Here's how the part is built. I have some questions about the finished solid (model axes, mm). A direction names the side the tool comes from. Round coordinates to 2 decimals unless told otherwise and drop trailing zeros. Write each loop counter-clockwise with the first axis right and the second up, starting at its lowest first coordinate (ties: lowest second). Pieces come first, ordered by that corner, then holes. Notation, with made-up numbers: (7.5, 77) -> (45.5, 77) arc R28 cw to (45.5, 104) -> close; hole circle Ø6 at (68, 74.25). An arc over 180 degrees is marked (long way). Put each result on its own line as item: value. Start each with the question number.
1) I want a section at B-B, the plane z = 46.99. List the corners of the cut face in (x, y) for me, then the cut area to 3 significant figures.
2) I want a section at D-D, the plane z = -16.51. Give the number of separate pieces and of enclosed holes in the cut face, then the cut area to 3 significant figures.
3) Will these pins go through, and if not, where does the flat tip stop? P1, Ø12, axis at y = 80.5, z = 34.5, coming from the -X side; P2, Ø0.9, axis at x = 1, z = 32.5, coming from the -Y side; P3, Ø0.8, axis at x = 1, z = 42.5, coming from the -Y side.
4) If I drill on line 1 along Y through (x, z) = (0.9, 46.99); line 2 along Y through (x, z) = (0.5, -18); line 3 along Y through (x, z) = (-3.25, 13.5), over which ranges is the centre line in solid material (lowest first)? Write a range as [from, to].
5) I want a section at C-C, the plane y = 12.7. List the corners of the cut face in (x, z) for me, then the cut area to 3 significant figures.
6) Which directions (+Z, -Z, +X, -X, +Y, -Y) give clear straight access to the entire face, cutting with the end or side of a thin tool? Please do faces 1 (the cylindrical face through (-0.955, 2.493, -4.952)), 2 (the flat face through (0.783, 25.561, -17.647)), 3 (the flat face through (-7, 1, 31.75)), 4 (the cylindrical face through (-11.62, 0.8, -2.73)), 5 (the cylindrical face through (0.2, 1.4, -5)).
7) I want a section at A-A, the plane y = 107.95. List the corners of the cut face in (x, z) for me, then the cut area to 3 significant figures.
8) We'd pull the mould along Z, two halves only. Please class faces 6 (the cylindrical face through (-12.943, 0.805, 17.205)), 7 (the flat face through (0.783, 46.246, 17.647)), 8 (the flat face through (0.3, 59.3, -40.64)), 9 (the cylindrical face through (0.805, 119.926, 30.986)): released by +Z, released by -Z, zero draft, split by the parting line, or undercut.
from build123d import *

# Parameters (mm, degrees)
SKETCH2_R                     = 14.2875
SKETCH2_R_2                   = 2.54
BOSS_EXTRUDE1_DEPTH           = 1.5875
SKETCH7_W                     = 1.5875
SKETCH7_H                     = 27.94
CUT_EXTRUDE1_DEPTH            = 0.00254
EDGE_FLANGE2_STRIP_W          = 12.7
EDGE_FLANGE2_STRIP_H          = 1.5875
EDGE_FLANGE2_STRIP_CUT_DEPTH  = 72.39
EDGE_FLANGE2_RELIEF_W         = 13.49375
EDGE_FLANGE2_RELIEF_H         = 0.79375
EDGE_FLANGE2_RELIEF_CUT_DEPTH = 1.5875
EDGE_FLANGE2_DEPTH            = 72.39
SKETCH14_R                    = 2.54
CUT_EXTRUDE2_DEPTH            = 1.5875
FILLET1_R                     = 2.54


# Sheet-metal steps are written as plain solids
with BuildPart() as part:
    # Sketch2 → Boss-Extrude1 (new body)
    with BuildSketch(Plane(origin=(0, 0, 0), x_dir=(0, 0, -1), z_dir=(1, 0, 0))):
        Polygon((-59.69, 95.25), (-59.69, 0), (40.64, 0), (40.64, 95.25), (40.64, 120.65), (-31.75, 120.65), (-31.75, 95.25), align=None)
        with Locations((0, 80.264)):
            Circle(SKETCH2_R, mode=Mode.SUBTRACT)
        with Locations((-46.99, 80.264)):
            Circle(SKETCH2_R_2, mode=Mode.SUBTRACT)
        with Locations((-46.99, 63.373)):
            Circle(SKETCH2_R_2, mode=Mode.SUBTRACT)
        with Locations((-17.272, 107.95)):
            Circle(SKETCH2_R_2, mode=Mode.SUBTRACT)
        with Locations((-2.794, 107.95)):
            Circle(SKETCH2_R_2, mode=Mode.SUBTRACT)
        with Locations((11.684, 107.95)):
            Circle(SKETCH2_R_2, mode=Mode.SUBTRACT)
        with Locations((26.162, 107.95)):
            Circle(SKETCH2_R_2, mode=Mode.SUBTRACT)
        with Locations((-46.99, 46.482)):
            Circle(SKETCH2_R_2, mode=Mode.SUBTRACT)
        with Locations((-46.99, 29.591)):
            Circle(SKETCH2_R_2, mode=Mode.SUBTRACT)
        with Locations((-46.99, 12.7)):
            Circle(SKETCH2_R_2, mode=Mode.SUBTRACT)
        with BuildLine():
            Line((-27.305, 64.866068321), (-8.255, 53.867545693))
            ThreePointArc((-8.255, 53.867545693), (-7.62, 52.76769343), (-8.255, 51.667841167))
            Line((-8.255, 51.667841167), (-27.305, 40.669318539))
            ThreePointArc((-27.305, 40.669318539), (-28.575, 40.669318539), (-29.21, 41.769170802))
            Line((-29.21, 41.769170802), (-29.21, 63.766216058))
            ThreePointArc((-29.21, 63.766216058), (-28.575, 64.866068321), (-27.305, 64.866068321))
        make_face(mode=Mode.SUBTRACT)
        with BuildLine():
            Line((-6.35, 43.235640486), (-6.35, 21.238595229))
            ThreePointArc((-6.35, 21.238595229), (-6.985, 20.138742967), (-8.255, 20.138742967))
            Line((-8.255, 20.138742967), (-27.305, 31.137265595))
            ThreePointArc((-27.305, 31.137265595), (-27.94, 32.237117857), (-27.305, 33.33697012))
            Line((-27.305, 33.33697012), (-8.255, 44.335492748))
            ThreePointArc((-8.255, 44.335492748), (-6.985, 44.335492748), (-6.35, 43.235640486))
        make_face(mode=Mode.SUBTRACT)
        with BuildLine():
            Line((8.255, 20.138742967), (27.305, 31.137265595))
            ThreePointArc((27.305, 31.137265595), (27.94, 32.237117857), (27.305, 33.33697012))
            Line((27.305, 33.33697012), (8.255, 44.335492748))
            ThreePointArc((8.255, 44.335492748), (6.985, 44.335492748), (6.35, 43.235640486))
            Line((6.35, 43.235640486), (6.35, 21.238595229))
            ThreePointArc((6.35, 21.238595229), (6.985, 20.138742967), (8.255, 20.138742967))
        make_face(mode=Mode.SUBTRACT)
        with BuildLine():
            Line((8.255, 51.667841167), (27.305, 40.669318539))
            ThreePointArc((27.305, 40.669318539), (28.575, 40.669318539), (29.21, 41.769170802))
            Line((29.21, 41.769170802), (29.21, 63.766216058))
            ThreePointArc((29.21, 63.766216058), (28.575, 64.866068321), (27.305, 64.866068321))
            Line((27.305, 64.866068321), (8.255, 53.867545693))
            ThreePointArc((8.255, 53.867545693), (7.62, 52.76769343), (8.255, 51.667841167))
        make_face(mode=Mode.SUBTRACT)
    extrude(amount=BOSS_EXTRUDE1_DEPTH)

    # Sketch7 → Cut-Extrude1 (cut)
    with BuildSketch(Plane(origin=(0, 0, 0), x_dir=(-1, 0, 0), z_dir=(0, -1, 0))):
        with Locations((-0.79375, -45.72)):
            Rectangle(SKETCH7_W, SKETCH7_H)
    extrude(amount=-CUT_EXTRUDE1_DEPTH, mode=Mode.SUBTRACT)

    # Edge-Flange2 strip (across the edge) → Edge-Flange2 strip cut (cut)
    with BuildSketch(Plane(origin=(0, 0, -40.64), x_dir=(0, 1, 0), z_dir=(0, 0, 1))):
        with Locations((-1.5875, -0.79375)):
            Rectangle(EDGE_FLANGE2_STRIP_W, EDGE_FLANGE2_STRIP_H)
    extrude(amount=EDGE_FLANGE2_STRIP_CUT_DEPTH, mode=Mode.SUBTRACT)

    # Edge-Flange2 relief (on the sheet) → Edge-Flange2 relief cut (cut)
    with BuildSketch(Plane(origin=(0, 4.7625, -40.64), x_dir=(0, 1, 0), z_dir=(-1, 0, 0))):
        with Locations((-5.953125, -72.786875)):
            Rectangle(EDGE_FLANGE2_RELIEF_W, EDGE_FLANGE2_RELIEF_H)
    extrude(amount=-EDGE_FLANGE2_RELIEF_CUT_DEPTH, mode=Mode.SUBTRACT)

    # Edge-Flange2 section (across the edge) → Edge-Flange2 (add)
    with BuildSketch(Plane(origin=(0, 0, -40.64), x_dir=(0, 1, 0), z_dir=(0, 0, 1))):
        with BuildLine():
            Line((0, 3.175), (0, 23.8125))
            Line((0, 23.8125), (1.5875, 23.8125))
            Line((1.5875, 23.8125), (1.5875, 3.175))
            ThreePointArc((1.5875, 3.175), (2.51743597, 0.92993597), (4.7625, 0))
            Line((4.7625, 0), (4.7625, -1.5875))
            ThreePointArc((4.7625, -1.5875), (1.394903955, -0.192596045), (0, 3.175))
        make_face()
    extrude(amount=EDGE_FLANGE2_DEPTH)

    # Sketch14 → Cut-Extrude2 (cut)
    with BuildSketch(Plane(origin=(0, 1.5875, 0), x_dir=(1, 0, 0), z_dir=(0, 1, 0))):
        with Locations(Location((-13.49375, 28.575, 0), (0, 0, 180))):
            Circle(SKETCH14_R)
        with Locations(Location((-13.49375, 16.51, 0), (0, 0, 180))):
            Circle(SKETCH14_R)
        with Locations(Location((-13.49375, 4.445, 0), (0, 0, 180))):
            Circle(SKETCH14_R)
        with Locations(Location((-13.49375, -7.62, 0), (0, 0, 180))):
            Circle(SKETCH14_R)
        with Locations(Location((-13.49375, -19.685, 0), (0, 0, 180))):
            Circle(SKETCH14_R)
    extrude(amount=-CUT_EXTRUDE2_DEPTH, mode=Mode.SUBTRACT)

    # Fillet1
    fillet1_edges = [part.edges().sort_by_distance(p)[0] for p in [
        (0.79375, 0.00254, 32.54375),
        (-23.8125, 0.79375, -40.64),
        (-23.8125, 0.79375, 31.75),
        (0.79375, 120.65, -40.64),
        (0.79375, 95.25, 59.69),
        (0.79375, 120.65, 31.75),
        (0.79375, 0.00254, 59.69),
    ]]
    fillet(fillet1_edges, radius=FILLET1_R)


solid = part.part
Findings:
1. outline: (0, 0) -> (1.59, 0) -> (1.59, 10.16) -> (0, 10.16) -> close; (0, 15.24) -> (1.59, 15.24) -> (1.59, 27.05) -> (0, 27.05) -> close; (0, 32.13) -> (1.59, 32.13) -> (1.59, 43.94) -> (0, 43.94) -> close; (0, 49.02) -> (1.59, 49.02) -> (1.59, 60.83) -> (0, 60.83) -> close; (0, 65.91) -> (1.59, 65.91) -> (1.59, 77.72) -> (0, 77.72) -> close; (0, 82.8) -> (1.59, 82.8) -> (1.59, 95.25) -> (0, 95.25) -> close
1. area: 111 mm2
2. separate pieces: 4
2. enclosed holes: 0
2. area: 177 mm2
3. P1: stops at x = 0
3. P2: stops at y = 1.16
3. P3: stops at y = 0
4. line 1: y = [0, 10.16], [15.24, 27.05], [32.13, 43.94], [49.02, 60.83], [65.91, 77.72], [82.8, 95.25]
4. line 2: y = [1.73, 25.77], [38.71, 46.04], [59.49, 120.65]
4. line 3: y = [0, 1.59]
5. outline: (0, -40.64) -> (1.59, -40.64) -> (1.59, 44.45) -> (0, 44.45) -> close; (0, 49.53) -> (1.59, 49.53) -> (1.59, 59.69) -> (0, 59.69) -> close
5. area: 151 mm2
6. face 1: +Z, -Z, -X, +Y
6. face 2: +X, -X
6. face 3: +X, -X, -Y
6. face 4: +Y, -Y
6. face 5: -Z, +X, -Y
7. outline: (0, -40.64) -> (1.59, -40.64) -> (1.59, -28.7) -> (0, -28.7) -> close; (0, -23.62) -> (1.59, -23.62) -> (1.59, -14.22) -> (0, -14.22) -> close; (0, -9.14) -> (1.59, -9.14) -> (1.59, 0.25) -> (0, 0.25) -> close; (0, 5.33) -> (1.59, 5.33) -> (1.59, 14.73) -> (0, 14.73) -> close; (0, 19.81) -> (1.59, 19.81) -> (1.59, 31.75) -> (0, 31.75) -> close
7. area: 82.7 mm2
8. face 6: undercut
8. face 7: undercut
8. face 8: released by -Z
8. face 9: released by +Z
